from build123d import *

# Parameters (mm, degrees)
SKETCH1_W           = 220
SKETCH1_H           = 230
BOSS_EXTRUDE1_DEPTH = 20
FILLET1_R           = 30
BOSS_EXTRUDE4_DEPTH = 10
CUT_EXTRUDE10_DEPTH = 17
SKETCH7_R           = 5
CUT_EXTRUDE3_DEPTH  = 31
SKETCH8_R           = 5
CUT_EXTRUDE4_DEPTH  = 30
SKETCH13_R          = 5
CUT_EXTRUDE5_DEPTH  = 30
CUT_EXTRUDE6_DEPTH  = 8.5
CUT_EXTRUDE7_DEPTH  = 8.5
CUT_EXTRUDE8_DEPTH  = 26.5
CUT_EXTRUDE9_DEPTH  = 31


with BuildPart() as part:
    # Sketch1 → Boss-Extrude1 (new body)
    with BuildSketch(Plane(origin=(0, 0, 0), x_dir=(1, 0, 0), z_dir=(0, 1, 0))):
        with Locations((110, 115)):
            Rectangle(SKETCH1_W, SKETCH1_H)
    extrude(amount=BOSS_EXTRUDE1_DEPTH)

    # Fillet1
    fillet1_edges = [part.edges().sort_by_distance(p)[0] for p in [
        (0, 10, -230),
        (220, 10, -230),
        (220, 10, 0),
        (0, 10, 0),
    ]]
    fillet(fillet1_edges, radius=FILLET1_R)

    # Sketch4 → Boss-Extrude4 (add)
    with BuildSketch(Plane(origin=(0, 0, 0), x_dir=(-1, 0, 0), z_dir=(0, -1, 0))):
        with BuildLine():
            Line((-210, 10), (-218.722813233, 10))
            ThreePointArc((-218.722813233, 10), (-206.201851746, -1.024184115), (-190, -5))
            Line((-190, -5), (-30, -5))
            ThreePointArc((-30, -5), (-13.798148254, -1.024184115), (-1.277186767, 10))
            Line((-1.277186767, 10), (-10, 10))
            Line((-10, 10), (-10, 15))
            Line((-10, 15), (1.622776602, 15))
            ThreePointArc((1.622776602, 15), (4.145257219, 22.312255892), (5, 30))
            Line((5, 30), (5, 40))
            Line((5, 40), (-10, 40))
            Line((-10, 40), (-10, 45))
            Line((-10, 45), (5, 45))
            Line((5, 45), (5, 70))
            Line((5, 70), (-10, 70))
            Line((-10, 70), (-10, 75))
            Line((-10, 75), (5, 75))
            Line((5, 75), (5, 100))
            Line((5, 100), (-10, 100))
            Line((-10, 100), (-10, 105))
            Line((-10, 105), (5, 105))
            Line((5, 105), (5, 130))
            Line((5, 130), (-10, 130))
            Line((-10, 130), (-10, 135))
            Line((-10, 135), (5, 135))
            Line((5, 135), (5, 160))
            Line((5, 160), (-10, 160))
            Line((-10, 160), (-10, 165))
            Line((-10, 165), (5, 165))
            Line((5, 165), (5, 190))
            Line((5, 190), (-10, 190))
            Line((-10, 190), (-10, 195))
            Line((-10, 195), (4.641016151, 195))
            ThreePointArc((4.641016151, 195), (4.058680517, 208.062647298), (-1.277186767, 220))
            Line((-1.277186767, 220), (-10, 220))
            Line((-10, 220), (-10, 228.722813233))
            ThreePointArc((-10, 228.722813233), (-19.519028269, 233.393850206), (-30, 235))
            Line((-30, 235), (-190, 235))
            ThreePointArc((-190, 235), (-200.480971731, 233.393850206), (-210, 228.722813233))
            Line((-210, 228.722813233), (-210, 220))
            Line((-210, 220), (-218.722813233, 220))
            ThreePointArc((-218.722813233, 220), (-224.058680517, 208.062647298), (-224.641016151, 195))
            Line((-224.641016151, 195), (-210, 195))
            Line((-210, 195), (-210, 190))
            Line((-210, 190), (-225, 190))
            Line((-225, 190), (-225, 165))
            Line((-225, 165), (-210, 165))
            Line((-210, 165), (-210, 160))
            Line((-210, 160), (-225, 160))
            Line((-225, 160), (-225, 135))
            Line((-225, 135), (-210, 135))
            Line((-210, 135), (-210, 130))
            Line((-210, 130), (-225, 130))
            Line((-225, 130), (-225, 105))
            Line((-225, 105), (-210, 105))
            Line((-210, 105), (-210, 100))
            Line((-210, 100), (-225, 100))
            Line((-225, 100), (-225, 75))
            Line((-225, 75), (-210, 75))
            Line((-210, 75), (-210, 70))
            Line((-210, 70), (-225, 70))
            Line((-225, 70), (-225, 45))
            Line((-225, 45), (-210, 45))
            Line((-210, 45), (-210, 40))
            Line((-210, 40), (-225, 40))
            Line((-225, 40), (-225, 30))
            ThreePointArc((-225, 30), (-224.145257219, 22.312255892), (-221.622776602, 15))
            Line((-221.622776602, 15), (-210, 15))
            Line((-210, 15), (-210, 10))
        make_face()
    extrude(amount=BOSS_EXTRUDE4_DEPTH)

    # Sketch20 → Cut-Extrude10 (cut)
    with BuildSketch(Plane(origin=(0, 20, 0), x_dir=(1, 0, 0), z_dir=(0, 1, 0))):
        with BuildLine():
            Line((215, 30), (215, 200))
            ThreePointArc((215, 200), (207.67766953, 217.67766953), (190, 225))
            Line((190, 225), (30, 225))
            ThreePointArc((30, 225), (12.32233047, 217.67766953), (5, 200))
            Line((5, 200), (5, 30))
            ThreePointArc((5, 30), (12.32233047, 12.32233047), (30, 5))
            Line((30, 5), (190, 5))
            ThreePointArc((190, 5), (207.67766953, 12.32233047), (215, 30))
        make_face()
    extrude(amount=-CUT_EXTRUDE10_DEPTH, mode=Mode.SUBTRACT)

    # Sketch7 → Cut-Extrude3 (cut, through all)
    with BuildSketch(Plane(origin=(0, -10, 0), x_dir=(-1, 0, 0), z_dir=(0, -1, 0))):
        with Locations((-42.5, 25)):
            Circle(SKETCH7_R)
        with Locations((-177.5, 25)):
            Circle(SKETCH7_R)
        with Locations((-177.5, 205)):
            Circle(SKETCH7_R)
        with Locations((-42.5, 205)):
            Circle(SKETCH7_R)
    extrude(amount=-CUT_EXTRUDE3_DEPTH, mode=Mode.SUBTRACT)

    # Sketch8 → Cut-Extrude4 (cut)
    with BuildSketch(Plane(origin=(0, 0, -230), x_dir=(-1, 0, 0), z_dir=(0, 0, -1))):
        with Locations((-150, 10)):
            Circle(SKETCH8_R)
        with Locations((-70, 10)):
            Circle(SKETCH8_R)
    extrude(amount=-CUT_EXTRUDE4_DEPTH, mode=Mode.SUBTRACT)

    # Sketch13 → Cut-Extrude5 (cut)
    with BuildSketch(Plane.XY):
        with Locations((70, 10)):
            Circle(SKETCH13_R)
        with Locations((150, 10)):
            Circle(SKETCH13_R)
    extrude(amount=-CUT_EXTRUDE5_DEPTH, mode=Mode.SUBTRACT)

    # Sketch17 → Cut-Extrude6 (cut)
    with BuildSketch(Plane.XY):
        Polygon((60.762395693, 10), (65.381197846, 2), (74.618802154, 2), (79.237604307, 10), (74.618802154, 18), (65.381197846, 18), align=None)
        Polygon((154.618802154, 18), (159.237604307, 10), (154.618802154, 2), (145.381197846, 2), (140.762395693, 10), (145.381197846, 18), align=None)
    extrude(amount=-CUT_EXTRUDE6_DEPTH, mode=Mode.SUBTRACT)

    # Sketch16 → Cut-Extrude7 (cut)
    with BuildSketch(Plane(origin=(0, 0, -230), x_dir=(-1, 0, 0), z_dir=(0, 0, -1))):
        Polygon((-159.237604307, 10), (-154.618802154, 2), (-145.381197846, 2), (-140.762395693, 10), (-145.381197846, 18), (-154.618802154, 18), align=None)
        Polygon((-65.381197846, 18), (-60.762395693, 10), (-65.381197846, 2), (-74.618802154, 2), (-79.237604307, 10), (-74.618802154, 18), align=None)
    extrude(amount=-CUT_EXTRUDE7_DEPTH, mode=Mode.SUBTRACT)

    # Sketch18 → Cut-Extrude8 (cut)
    with BuildSketch(Plane(origin=(0, 20, 0), x_dir=(1, 0, 0), z_dir=(0, 1, 0))):
        Polygon((42.5, 195.762395693), (50.5, 200.381197846), (50.5, 209.618802154), (42.5, 214.237604307), (34.5, 209.618802154), (34.5, 200.381197846), align=None)
        Polygon((185.5, 200.381197846), (177.5, 195.762395693), (169.5, 200.381197846), (169.5, 209.618802154), (177.5, 214.237604307), (185.5, 209.618802154), align=None)
        Polygon((185.5, 20.381197846), (185.5, 29.618802154), (177.5, 34.237604307), (169.5, 29.618802154), (169.5, 20.381197846), (177.5, 15.762395693), align=None)
        Polygon((34.5, 29.618802154), (42.5, 34.237604307), (50.5, 29.618802154), (50.5, 20.381197846), (42.5, 15.762395693), (34.5, 20.381197846), align=None)
    extrude(amount=-CUT_EXTRUDE8_DEPTH, mode=Mode.SUBTRACT)

    # Sketch19 → Cut-Extrude9 (cut, through all)
    with BuildSketch(Plane(origin=(0, 20, 0), x_dir=(1, 0, 0), z_dir=(0, 1, 0))):
        with BuildLine():
            Line((85, 185), (135, 185))
            ThreePointArc((135, 185), (145, 175), (135, 165))
            Line((135, 165), (85, 165))
            ThreePointArc((85, 165), (75, 175), (85, 185))
        make_face()
    extrude(amount=-CUT_EXTRUDE9_DEPTH, mode=Mode.SUBTRACT)


solid = part.part
Read the model definition and answer for the solid it produces. Units are mm, in the model's axes. A direction names the side the tool comes from. Give positions to 0.01 mm unless a question says otherwise; leave off trailing zeros. Write each loop counter-clockwise with the first axis right and the second up, starting at its lowest first coordinate (ties: lowest second). Pieces come first, ordered by that corner, then holes. Notation, with made-up numbers: M 81,-28.75 L 110,-28.75 A18 cw 110,-13.75 Z; hole C 83.5,1.5 d8. An arc over 180 degrees is marked long. One line per item, written item: value. Start each with the question number.
(1) Find section A-A (x = 100.5). Determine the outline of the cut face in (y, z).
(2) Find the intervals of material crossed by line 1 (Z direction, x = 42.5, y = -8.1); line 2 (X direction, y = -8.65, z = -25); line 3 (Z direction, x = 82.5, y = 4.5), in increasing order.
(3) Determine the mould class of faces 1 (the flat face through (225, -5, -178)), 2 (the flat face through (156.961, 6.056, -2.302)) for opening direction Y: pulls with the +Y half, pulls with the -Y half, needs draft (parallel to the pull), parting line crosses it, or undercut.
(4) Flat-ended cylindrical pins translate along their axes: pin 1 Ø1.5 at (y, z) = (7.5, -208.5) entering from -X; pin 2 Ø4 at (x, z) = (83.5, -195.5) entering from +Y; pin 3 Ø7 at (x, y) = (6, -3.5) entering from -Z. Find the tip coordinate at first contact, or state that the pin passes through.
(5) Find section C-C (y = 6.75). Give the number of separate pieces and of enclosed holes in the cut face, plus the area to 3 significant figures.
(6) Find section B-B (z = -175). Determine the outline of the cut face in (x, y).
(7) A tool of negligible diameter and unlimited length cuts with its end or side. For faces 3 (the flat face through (143.104, 5.944, -227.698)), 4 (the flat face through (109, 10, -230)), 5 (the flat face through (4, -5, -15)), 6 (the cylindrical face through (145, -3, -175)), 7 (the flat face through (169.5, -2, -205)), from which of +Z, -Z, +X, -X, +Y, -Y can it reach the whole face along a straight path? Write none if from no direction.
(8) Find section D-D (z = -122.5). Determine the outline of the cut face in (x, y), plus the area to 3 significant figures.
Results below:
1. outline: M -10,-235 L 0,-235 L 0,-230 L 20,-230 L 20,-225 L 3,-225 L 3,-185 L -10,-185 Z; M -10,-165 L 3,-165 L 3,-5 L 20,-5 L 20,0 L 0,0 L 0,5 L -10,5 Z
2. line 1: z = -235 to -210, -200 to -30, -20 to 5
2. line 2: x = -4.64 to 37.5, 47.5 to 172.5, 182.5 to 224.64
2. line 3: z = -230 to -225, -5 to 0
3. face 1: needs draft
3. face 2: undercut
4. pin 1: stops at x = 1.02
4. pin 2: stops at y = 3
4. pin 3: stops at z = -220
5. separate pieces: 4
5. enclosed holes: 0
5. area: 3,870 mm^2
6. outline: M -5,-10 L 75,-10 L 75,3 L 5,3 L 5,20 L 0,20 L 0,0 L -5,0 Z; M 145,-10 L 225,-10 L 225,0 L 220,0 L 220,20 L 215,20 L 215,3 L 145,3 Z
7. face 3: -Z
7. face 4: -Z, +X, -X, +Y
7. face 5: -X, -Y
7. face 6: +Y, -Y
7. face 7: +Y
8. outline: M -5,-10 L 225,-10 L 225,0 L 220,0 L 220,20 L 215,20 L 215,3 L 5,3 L 5,20 L 0,20 L 0,0 L -5,0 Z
8. area: 3,130 mm^2
